from build123d import *

# Parameters (mm, degrees)
F1_DEPTH = 10.16
F2_DEPTH = 10.16


with BuildPart() as f1:
    # F0 (on Front) → F1 (new body)
    with BuildSketch(Plane.XZ):
        with BuildLine():
            Line((5.086044, 6.534736), (-5.073956, 6.534736))
            Line((-5.073956, 6.534736), (-5.073956, 0.567228))
            ThreePointArc((-5.073956, 0.567228), (0.060908, 5.1052), (5.086044, 0.446012))
            Line((5.086044, 0.446012), (5.086044, 6.534736))
        make_face()
    extrude(amount=F1_DEPTH)

    # F0 (on Front) → F2 (join)
    with BuildSketch(Plane.XZ):
        with BuildLine():
            ThreePointArc((5.086044, 0.446012), (0.060908, 5.1052), (-5.073956, 0.567228))
            ThreePointArc((-5.073956, 0.567228), (-0.284054, -5.097655), (5.105563, 0))
            ThreePointArc((5.105563, 0), (5.100681, 0.223219), (5.086044, 0.446012))
        make_face()
    extrude(amount=F2_DEPTH)


solid = f1.part
Here's how the part is built. I have some questions about the finished solid (model axes, mm). A direction names the side the tool comes from. Round coordinates to 2 decimals unless told otherwise and drop trailing zeros. Write each loop counter-clockwise with the first axis right and the second up, starting at its lowest first coordinate (ties: lowest second). Pieces come first, ordered by that corner, then holes.
1. Suppose I cut it at C-C (x = -2). List the corners of the cut face in (y, z) for me, and give its area (3 significant figures).
2. Suppose I cut it at B-B (z = -4). List the corners of the cut face in (x, y) for me, and give its area (3 significant figures).
3. Suppose I cut it at A-A (y = -5). List the corners of the cut face in (x, z) for me, and give its area (3 significant figures).
4. For faces 1 (the flat face through (0, -10.16, 1)), 2 (the flat face through (5.086, -5, 3)), 3 (the flat face through (-5.074, -5, 4)), which set-ups out of +Z, -Z, +X, -X, +Y, -Y let a thin tool reach every point of the face, with its end or its side?
5. Will these pins go through, and if not, where does the flat tip stop? pin 1 Ø3 at (y, z) = (-5, 2.5) entering from +X; pin 2 Ø1 at (y, z) = (-5, 4) entering from -X; pin 3 Ø1.5 at (x, z) = (-2, 1) entering from +Y; pin 4 Ø2 at (y, z) = (-3, -2.5) entering from -X.
6. I need wall thicknesses on L1, parallel to X at y = -4, z = 2.5; L2, parallel to Z at x = 3.5, y = -4.75; L3, parallel to X at y = -6.25, z = -1.75. Which ranges of each line are inside material? Lowest first, please.
Answer sheet:
1. outline: (-10.16, -4.7) - (0, -4.7) - (0, 6.53) - (-10.16, 6.53) - close
1. area: 114 mm2
2. outline: (-3.17, -10.16) - (3.17, -10.16) - (3.17, 0) - (-3.17, 0) - close
2. area: 64.5 mm2
3. outline: (-5.07, 0.57) arc R5.11 ccw (long way) to (5.11, 0) arc R5.11 ccw to (5.09, 0.45) - (5.09, 6.53) - (-5.07, 6.53) - close
3. area: 107 mm2
4. face 1: +Z, -Z, +X, -X, -Y
4. face 2: +Z, +X, +Y, -Y
4. face 3: +Z, -X, +Y, -Y
5. pin 1: stops at x = 5.09
5. pin 2: stops at x = -5.07
5. pin 3: stops at y = 0
5. pin 4: stops at x = -4.88
6. L1: x = -5.07 to 5.09
6. L2: z = -3.72 to 6.53
6. L3: x = -4.8 to 4.8
